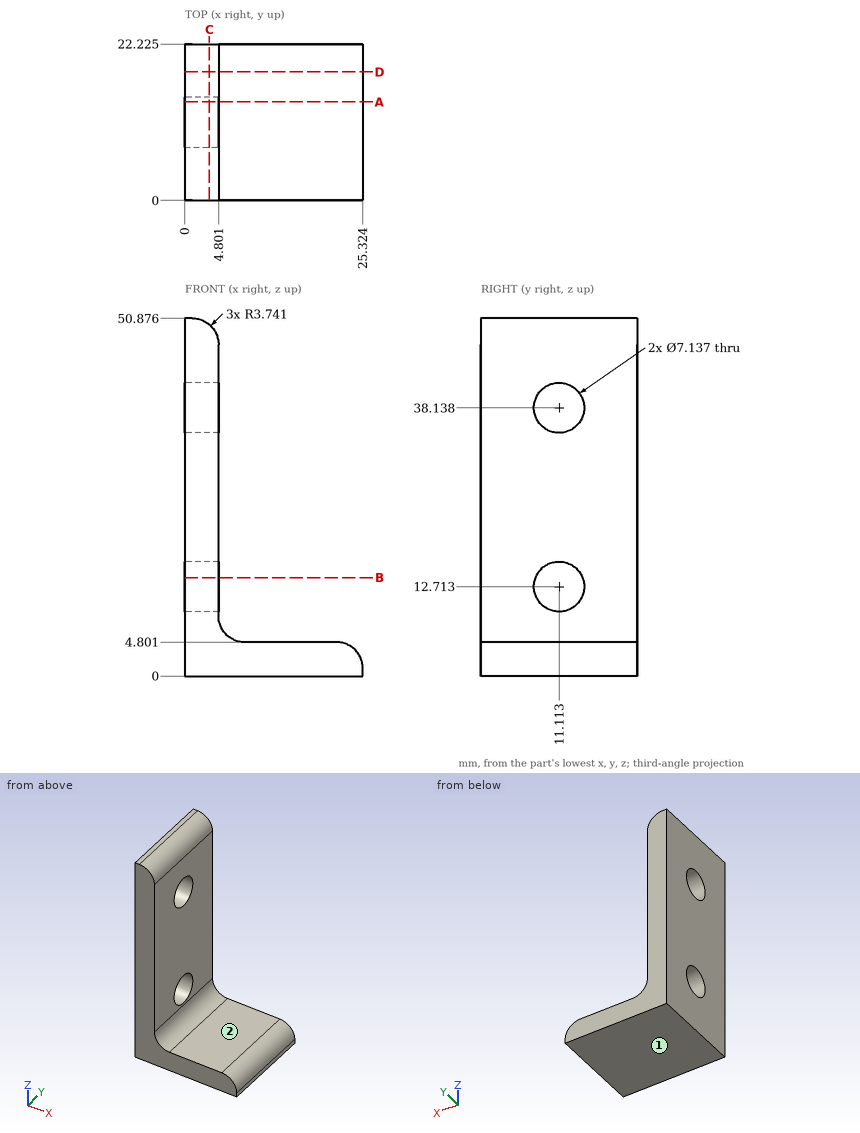
The figure shows three views and two pictorial views of one solid part (mm, origin at its lowest corner). Answer the questions. A direction names the side the tool comes from. Give positions to 0.01 mm unless a question says otherwise; leave off trailing zeros. Write each loop counter-clockwise with the first axis right and the second up, starting at its lowest first coordinate (ties: lowest second). Pieces come first, ordered by that corner, then holes. Notation, with made-up numbers: M -39,-25 L 10,-25 A6 cw 10,-19 Z; hole C 72.25,-20 d10. An arc over 180 degrees is marked long. One line per item, written item: value. Start each with the question number.
(1) Find section D-D (y = 18.25). Determine the outline of the cut face in (x, z) (1 decimal), plus the area to 3 significant figures.
(2) Find section B-B (z = 14). Determine the outline of the cut face in (x, y) (1 decimal).
(3) Find the intervals of material crossed by line 1 (X direction, y = 5.75, z = 12.5); line 2 (X direction, y = 9.5, z = 3.5), in increasing order.
(4) A tool of negligible diameter and unlimited length cuts with its end or side. For the marked faces 1 and 2, from which of +Z, -Z, +X, -X, +Y, -Y can it reach the whole face along a straight path? Write none if from no direction.
(5) Find section A-A (y = 14). Determine the outline of the cut face in (x, z) (1 decimal).
(6) Find section C-C (x = 3.5). Determine the outline of the cut face in (y, z) (1 decimal), plus the area to 3 significant figures.
(7) Flat-ended cylindrical pins translate along their axes: pin 1 Ø9.5 at (y, z) = (11.11, 12.71) entering from +X; pin 2 Ø6.5 at (x, y) = (13.5, 14.5) entering from +Z; pin 3 Ø6.5 at (y, z) = (11.11, 38.14) entering from +X. Find the tip coordinate at first contact, or state that the pin passes through.
Results below:
1. outline: M 0,0 L 25.3,0 L 25.3,1.1 A3.7 ccw 21.6,4.8 L 8.5,4.8 A3.7 cw 4.8,8.5 L 4.8,47.1 A3.7 ccw 1.1,50.9 L 0,50.9 Z
1. area: 340 mm^2
2. outline: M 0,0 L 4.8,0 L 4.8,7.8 L 0,7.8 Z; M 0,14.4 L 4.8,14.4 L 4.8,22.2 L 0,22.2 Z
3. line 1: x = 0 to 4.8
3. line 2: x = 0 to 24.42
4. face 1: -Z, +X, -X, +Y, -Y
4. face 2: +Z, +X, +Y, -Y
5. outline: M 0,0 L 25.3,0 L 25.3,1.1 A3.7 ccw 21.6,4.8 L 8.5,4.8 A3.7 cw 4.8,8.5 L 4.8,10.6 L 0,10.6 Z; M 0,14.8 L 4.8,14.8 L 4.8,36 L 0,36 Z; M 0,40.2 L 4.8,40.2 L 4.8,47.1 A3.7 ccw 1.1,50.9 L 0,50.9 Z
6. outline: M 0,0 L 22.2,0 L 22.2,50 L 0,50 Z; hole C 11.1,12.7 d7.1; hole C 11.1,38.1 d7.1
6. area: 1,030 mm^2
7. pin 1: stops at x = 4.85
7. pin 2: stops at z = 4.8
7. pin 3: passes through
